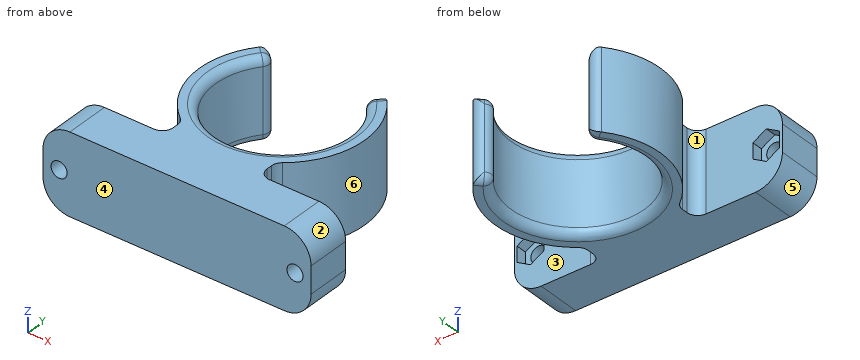
```python
from build123d import *

# Parameters (mm, degrees)
RESSALTO_EXTRUS_O1_DEPTH = 15
ESBO_O3_R                = 1.5
CORTE_EXTRUS_O1_DEPTH    = 8.219669914
CORTE_EXTRUS_O2_DEPTH    = 2
FILETE1_R                = 1.5
FILETE2_R                = 2
FILETE3_R                = 5


with BuildPart() as part:
    # Esboço2 → Ressalto-extrusão1 (new body)
    with BuildSketch(Plane.XY):
        with BuildLine():
            Line((-25, -4.380330086), (-25, -12.6))
            Line((-25, -12.6), (25, -12.6))
            Line((25, -12.6), (25, -4.380330086))
            Line((25, -4.380330086), (8.768124087, -4.380330086))
            Line((8.768124087, -4.380330086), (8.768124087, -0.260173774))
            ThreePointArc((8.768124087, -0.260173774), (15.361943152, 11.318009898), (10.456147688, 23.706147688))
            Line((10.456147688, 23.706147688), (8.332817936, 21.582817936))
            ThreePointArc((8.332817936, 21.582817936), (0.30060873, 0.00364431), (-8.768124087, 21.168124087))
            Line((-8.768124087, 21.168124087), (-10.88944443, 23.28944443))
            ThreePointArc((-10.88944443, 23.28944443), (-15.337898467, 11.018381166), (-8.768124087, -0.260173774))
            Line((-8.768124087, -0.260173774), (-8.768124087, -4.380330086))
            Line((-8.768124087, -4.380330086), (-25, -4.380330086))
        make_face()
    extrude(amount=RESSALTO_EXTRUS_O1_DEPTH)

    # Esboço3 → Corte-extrusão1 (cut)
    with BuildSketch(Plane(origin=(0, -4.380330086, 0), x_dir=(1, 0, 0), z_dir=(0, 1, 0))):
        with Locations(Location((22, -7.5, 0), (0, 0, 270))):
            Circle(ESBO_O3_R)
        with Locations(Location((-22, -7.5, 0), (0, 0, 180))):
            Circle(ESBO_O3_R)
    extrude(amount=-CORTE_EXTRUS_O1_DEPTH, mode=Mode.SUBTRACT)

    # Esboço5 → Corte-extrusão2 (cut)
    with BuildSketch(Plane(origin=(0, -4.380330086, 0), x_dir=(1, 0, 0), z_dir=(0, 1, 0))):
        Polygon((22, -4.613248654), (19.5, -6.056624327), (19.5, -8.943375673), (22, -10.386751346), (24.5, -8.943375673), (24.5, -6.056624327), align=None)
        Polygon((-24.5, -6.056624327), (-22, -4.613248654), (-19.5, -6.056624327), (-19.5, -8.943375673), (-22, -10.386751346), (-24.5, -8.943375673), align=None)
    extrude(amount=-CORTE_EXTRUS_O2_DEPTH, mode=Mode.SUBTRACT)

    # Filete1
    filete1_edges = [part.edges().sort_by_distance(p)[0] for p in [
        (9.394482812, 22.644482812, 15),
        (-9.828784258, 22.228784258, 0),
        (0.30060873, 0.00364431, 0),
        (9.394482812, 22.644482812, 0),
        (0.30060873, 0.00364431, 15),
        (-10.88944443, 23.28944443, 7.5),
        (-8.768124087, 21.168124087, 7.5),
        (8.332817936, 21.582817936, 7.5),
        (10.456147688, 23.706147688, 7.5),
        (-9.828784258, 22.228784258, 15),
    ]]
    fillet(filete1_edges, radius=FILETE1_R - 0.0001)  # a hair under: the kernel refuses the full size

    # Filete2
    filete2_edges = [part.edges().sort_by_distance(p)[0] for p in [
        (8.768124087, -4.380330086, 7.5),
        (-8.768124087, -4.380330086, 7.5),
        (-8.768124087, -0.260173774, 7.5),
        (8.768124087, -0.260173774, 7.5),
    ]]
    fillet(filete2_edges, radius=FILETE2_R)

    # Filete3
    filete3_edges = [part.edges().sort_by_distance(p)[0] for p in [
        (25, -8.490165043, 0),
        (-25, -8.490165043, 0),
        (-25, -8.490165043, 15),
        (25, -8.490165043, 15),
    ]]
    fillet(filete3_edges, radius=FILETE3_R)


solid = part.part
```
Input: part model. Units: mm. Frame: model coordinates. Face numbers are marked on the shaded views. A direction names the side the tool comes from. Give positions to 0.01 mm unless a question says otherwise; leave off trailing zeros. Order: outer loops, then holes, each group sorted by start corner. A loop starts at its lowest first (then second) coordinate and runs counter-clockwise, first axis right, second up. Notation, with made-up numbers: (50.25, 70.25) - (78.25, 70.25) arc R23 cw to (78.25, 85.25) - close; hole circle Ø7 at (72.25, -31). An arc over 180 degrees is marked (long way). Use a Markdown table: item, result.
(1) Section query D-D (z = 6.75). State how many separate pieces and enclosed holes the cut face has, then the cut area to 3 significant figures.
Computed values:
| item | result |
|---|---|
| separate pieces | 3 |
| enclosed holes | 0 |
| area | 597 mm2 |
(2) Access query for the marked faces 1, 2 and 3. Directions: +Z, -Z, +X, -X, +Y, -Y. A direction counts if a zero-diameter tool reaches every point of the face in a straight line with its end or side. Return the directions, or none.
Computed values:
| item | result |
|---|---|
| face 1 | +Z, -Z, -X |
| face 2 | +Z, +X, +Y, -Y |
| face 3 | +Z, -Z, +X |
(3) Pin query (flat end, axial travel): pin 1 (4.5 mm diameter, centred on x = 20.5, z = 5.5, fed in from +Y); pin 2 (2.5 mm diameter, centred on x = 22, z = 7.5, fed in from -Y); pin 3 (1.2 mm diameter, centred on y = -2, z = 7, fed in from +X); pin 4 (5 mm diameter, centred on x = -2, y = 1.5, fed in from +Z). Return the tip coordinate at first contact, or that it passes through.
Computed values:
| item | result |
|---|---|
| pin 1 | stops at y = -4.38 |
| pin 2 | passes through |
| pin 3 | stops at x = 8.78 |
| pin 4 | stops at z = 14.97 |
(4) Section query A-A (y = -9). Output: boundary loops of the cut face in (x, z).
Computed values:
| item | result |
|---|---|
| outline | (-25, 5) arc R5 ccw to (-20, 0) - (20, 0) arc R5 ccw to (25, 5) - (25, 10) arc R5 ccw to (20, 15) - (-20, 15) arc R5 ccw to (-25, 10) - close; hole circle Ø3 at (-22, 7.5); hole circle Ø3 at (22, 7.5) |
(5) Section query B-B (x = 16.5). Output: boundary loops of the cut face in (y, z), then the cut area to 3 significant figures.
Computed values:
| item | result |
|---|---|
| outline | (-12.6, 0) - (-4.38, 0) - (-4.38, 15) - (-12.6, 15) - close |
| area | 123 mm2 |
(6) Line query: line 1 (Y direction, x = -9.5, z = 4); line 2 (X direction, y = 12.4, z = 4.25); line 3 (Y direction, x = 0, z = 8.5). Output: solid intervals per line, ascending. Write a range as from..to.
Computed values:
| item | result |
|---|---|
| line 1 | y = -12.6..-3.93, 0.28..4.43, 20.42..21.8 |
| line 2 | x = -15.4..-12.4, 12.4..15.4 |
| line 3 | y = -12.6..0 |
(7) Draft query along Y for the marked faces 4, 5 and 6. Return one class per face: released by +Y, released by -Y, zero draft, split by the parting line, or undercut.
Computed values:
| item | result |
|---|---|
| face 4 | released by -Y |
| face 5 | zero draft |
| face 6 | undercut |
